from build123d import *
from OCP.BRepFilletAPI import BRepFilletAPI_MakeChamfer

# Parameters (mm, degrees)
SKETCH1_W           = 87
SKETCH1_H           = 52
BOSS_EXTRUDE1_DEPTH = 29.5
BOSS_EXTRUDE1_TAPER = 2
CHAMFER1_SIZE       = 2
CHAMFER1_SIZE2      = 2.002440407
CHAMFER2_SIZE       = 2
CHAMFER2_SIZE2      = 2.073631911
CHAMFER2_SIZE2_2    = 2.106466142
SKETCH2_R           = 0.5
SKETCH2_R_2         = 1
BOSS_EXTRUDE2_DEPTH = 3.5


with BuildPart() as part:
    # Sketch1 → Boss-Extrude1 (new body)
    with BuildSketch(Plane.XY):
        Rectangle(SKETCH1_W, SKETCH1_H)
    extrude(amount=BOSS_EXTRUDE1_DEPTH, taper=BOSS_EXTRUDE1_TAPER)

    # Chamfer1: one chamfer whose edges measure the first distance from different faces: ONE call of the kernel's chamfer builder (chamfer() names one face for all edges)
    chamfer1_edges_1 = [part.edges().sort_by_distance(p)[0] for p in [
        (42.98491865, -25.48491865, 14.75),
    ]]
    chamfer1_side_1 = [part.faces().sort_by_distance(p)[0] for p in [
        (0, -25.486976029, 14.691084376),
    ]]
    chamfer1_edges_2 = [part.edges().sort_by_distance(p)[0] for p in [
        (-42.984918188, -25.484918188, 14.750013228),
    ]]
    chamfer1_side_2 = [part.faces().sort_by_distance(p)[0] for p in [
        (-42.988388791, 0, 14.650628158),
    ]]
    chamfer1_edges_3 = [part.edges().sort_by_distance(p)[0] for p in [
        (-42.98491865, 25.48491865, 14.75),
    ]]
    chamfer1_side_3 = [part.faces().sort_by_distance(p)[0] for p in [
        (0, 25.486976029, 14.691084376),
    ]]
    chamfer1_edges_4 = [part.edges().sort_by_distance(p)[0] for p in [
        (42.98491865, 25.48491865, 14.75),
    ]]
    chamfer1_side_4 = [part.faces().sort_by_distance(p)[0] for p in [
        (42.988388791, 0, 14.650628158),
    ]]
    chamfer1 = BRepFilletAPI_MakeChamfer(part.part.solid().wrapped)
    for e in chamfer1_edges_1:
        chamfer1.Add(CHAMFER1_SIZE, CHAMFER1_SIZE2, e.wrapped, chamfer1_side_1[0].wrapped)  # the first distance lies on this face
    for e in chamfer1_edges_2:
        chamfer1.Add(CHAMFER1_SIZE, CHAMFER1_SIZE2, e.wrapped, chamfer1_side_2[0].wrapped)  # the first distance lies on this face
    for e in chamfer1_edges_3:
        chamfer1.Add(CHAMFER1_SIZE, CHAMFER1_SIZE2, e.wrapped, chamfer1_side_3[0].wrapped)  # the first distance lies on this face
    for e in chamfer1_edges_4:
        chamfer1.Add(CHAMFER1_SIZE, CHAMFER1_SIZE2, e.wrapped, chamfer1_side_4[0].wrapped)  # the first distance lies on this face
    add(Compound.cast(chamfer1.Shape()), mode=Mode.REPLACE)

    # Chamfer2: one chamfer whose edges measure the first distance from different faces: ONE call of the kernel's chamfer builder (chamfer() names one face for all edges)
    chamfer2_edges_1 = [part.edges().sort_by_distance(p)[0] for p in [
        (42.4698373, 0.001220947, 29.5),
    ]]
    chamfer2_side_1 = [part.faces().sort_by_distance(p)[0] for p in [
        (42.988684703, 0.001220947, 14.642154351),
    ]]
    chamfer2_edges_2 = [part.edges().sort_by_distance(p)[0] for p in [
        (0.001220947, -24.9698373, 29.5),
    ]]
    chamfer2_side_2 = [part.faces().sort_by_distance(p)[0] for p in [
        (0.001220947, -25.487076554, 14.688205709),
    ]]
    chamfer2_edges_3 = [part.edges().sort_by_distance(p)[0] for p in [
        (-0.001220947, 24.9698373, 29.5),
    ]]
    chamfer2_side_3 = [part.faces().sort_by_distance(p)[0] for p in [
        (-0.001220947, 25.487076554, 14.688205709),
    ]]
    chamfer2_edges_4 = [part.edges().sort_by_distance(p)[0] for p in [
        (-42.4698373, -0.001220947, 29.5),
    ]]
    chamfer2_side_4 = [part.faces().sort_by_distance(p)[0] for p in [
        (-42.988684703, -0.001220947, 14.642154351),
    ]]
    chamfer2_edges_5 = [part.edges().sort_by_distance(p)[0] for p in [
        (-41.469228498, 23.968007551, 29.5),
    ]]
    chamfer2_side_5 = [part.faces().sort_by_distance(p)[0] for p in [
        (-41.984309848, 24.483088901, 14.75),
    ]]
    chamfer2_edges_6 = [part.edges().sort_by_distance(p)[0] for p in [
        (-41.468007551, -23.969228498, 29.5),
    ]]
    chamfer2_side_6 = [part.faces().sort_by_distance(p)[0] for p in [
        (-41.983088901, -24.484309848, 14.75),
    ]]
    chamfer2_edges_7 = [part.edges().sort_by_distance(p)[0] for p in [
        (41.468007551, 23.969228498, 29.5),
    ]]
    chamfer2_side_7 = [part.faces().sort_by_distance(p)[0] for p in [
        (41.983088901, 24.484309848, 14.75),
    ]]
    chamfer2_edges_8 = [part.edges().sort_by_distance(p)[0] for p in [
        (41.469228498, -23.968007551, 29.5),
    ]]
    chamfer2_side_8 = [part.faces().sort_by_distance(p)[0] for p in [
        (41.984309848, -24.483088901, 14.75),
    ]]
    chamfer2 = BRepFilletAPI_MakeChamfer(part.part.solid().wrapped)
    for e in chamfer2_edges_1:
        chamfer2.Add(CHAMFER2_SIZE, CHAMFER2_SIZE2, e.wrapped, chamfer2_side_1[0].wrapped)  # the first distance lies on this face
    for e in chamfer2_edges_2:
        chamfer2.Add(CHAMFER2_SIZE, CHAMFER2_SIZE2, e.wrapped, chamfer2_side_2[0].wrapped)  # the first distance lies on this face
    for e in chamfer2_edges_3:
        chamfer2.Add(CHAMFER2_SIZE, CHAMFER2_SIZE2, e.wrapped, chamfer2_side_3[0].wrapped)  # the first distance lies on this face
    for e in chamfer2_edges_4:
        chamfer2.Add(CHAMFER2_SIZE, CHAMFER2_SIZE2, e.wrapped, chamfer2_side_4[0].wrapped)  # the first distance lies on this face
    for e in chamfer2_edges_5:
        chamfer2.Add(CHAMFER2_SIZE, CHAMFER2_SIZE2_2, e.wrapped, chamfer2_side_5[0].wrapped)  # the first distance lies on this face
    for e in chamfer2_edges_6:
        chamfer2.Add(CHAMFER2_SIZE, CHAMFER2_SIZE2_2, e.wrapped, chamfer2_side_6[0].wrapped)  # the first distance lies on this face
    for e in chamfer2_edges_7:
        chamfer2.Add(CHAMFER2_SIZE, CHAMFER2_SIZE2_2, e.wrapped, chamfer2_side_7[0].wrapped)  # the first distance lies on this face
    for e in chamfer2_edges_8:
        chamfer2.Add(CHAMFER2_SIZE, CHAMFER2_SIZE2_2, e.wrapped, chamfer2_side_8[0].wrapped)  # the first distance lies on this face
    add(Compound.cast(chamfer2.Shape()), mode=Mode.REPLACE)

    # Sketch2 → Boss-Extrude2 (add)
    with BuildSketch(Plane(origin=(0, 0, 0), x_dir=(-1, 0, 0), z_dir=(0, 0, -1))):
        with Locations(Location((38.2, 21, 0), (0, 0, 180))):
            Circle(SKETCH2_R)
        with Locations(Location((38.2, 14.25, 0), (0, 0, 180))):
            Circle(SKETCH2_R)
        with Locations(Location((-37.8, -14.75, 0), (0, 0, 180))):
            Circle(SKETCH2_R_2)
        with Locations(Location((-37.8, -20.25, 0), (0, 0, 180))):
            Circle(SKETCH2_R_2)
    extrude(amount=BOSS_EXTRUDE2_DEPTH)


solid = part.part
Read the model definition and answer for the solid it produces. Units are mm, in the model's axes. Round coordinates to 2 decimals unless told otherwise and drop trailing zeros. Loops run counter-clockwise (first coordinate to the right, second up) from the corner with the lowest first, then second, coordinate; pieces in that order, holes last.
Q1. Section A-A on y = -2.5 is taken. Write down the section's boundary in (x, z).
Q2. Section C-C on z = 25 is taken. Write down the section's boundary in (x, y), and give its area (3 significant figures).
Q3. Each of these flat-tipped pins is pushed along its axis until it touches: pin 1 (1.5 mm diameter, centred on x = 17.5, z = 16, fed in from -Y); pin 2 (6 mm diameter, centred on y = -2.5, z = 12.5, fed in from -X); pin 3 (4 mm diameter, centred on y = -9, z = 11, fed in from +X). Where does it stop, or does it pass through?
Q4. Section B-B on x = -20 is taken. Write down the section's boundary in (y, z), and give its area (3 significant figures).
Q5. Consider probe 1 along Z at (x, y) = (-15.5, 14); probe 2 along Y at (x, z) = (-39, 27); probe 3 along X at (y, z) = (-12.5, 27). Determine where each line is inside the solid, lowest interval first.
Q6. Determine the mould class of faces 1 (the face through (40.935, 23.407, 28.293)), 2 (the face through (40.907, -23.435, 28.293)), 3 (the face through (37.583, -13.774, -1.726)) for opening direction Y: released by +Y, released by -Y, zero draft, split by the parting line, or undercut.
Q7. Section D-D on y = -20.25 is taken. Write down the section's boundary in (x, z), and give its area (3 significant figures).
Output:
1. outline: (-43.5, 0) - (43.5, 0) - (42.54, 27.5) - (40.4, 29.5) - (-40.4, 29.5) - (-42.54, 27.5) - close
2. outline: (-42.63, -23.13) - (-40.62, -25.13) - (40.63, -25.13) - (42.63, -23.12) - (42.63, 23.13) - (40.62, 25.13) - (-40.63, 25.13) - (-42.63, 23.12) - close
2. area: 4,280 mm2
3. pin 1: stops at y = -25.47
3. pin 2: stops at x = -43.17
3. pin 3: stops at x = 43.19
4. outline: (-26, 0) - (26, 0) - (25.04, 27.5) - (22.9, 29.5) - (-22.9, 29.5) - (-25.04, 27.5) - close
4. area: 1,500 mm2
5. probe 1: z = 0 to 29.5
5. probe 2: y = -25.06 to 25.06
5. probe 3: x = -42.56 to 42.56
6. face 1: released by +Y
6. face 2: released by -Y
6. face 3: undercut
7. outline: (-43.5, 0) - (36.8, 0) - (36.8, -3.5) - (38.8, -3.5) - (38.8, 0) - (43.5, 0) - (42.54, 27.5) - (40.4, 29.5) - (-40.4, 29.5) - (-42.54, 27.5) - close
7. area: 2,540 mm2
